Verification items for the finished model (mm, model axes). A direction names the side the tool comes from. Give positions to 0.01 mm unless a question says otherwise; leave off trailing zeros. Order: outer loops, then holes, each group sorted by start corner. A loop starts at its lowest first (then second) coordinate and runs counter-clockwise, first axis right, second up. Notation, with made-up numbers: M 7.5,-5 L 41.5,-5 A14 ccw 41.5,-1 Z; hole C -20,17.25 d5. An arc over 180 degrees is marked long. Answer as a JSON object with one key per item and string values.
```python
from build123d import *

# Parameters (mm, degrees)
F0_R     = 16
F1_DEPTH = 25
F3_R     = 7.5
F4_DEPTH = 20
F5_T     = -2
F6_R     = 3


with BuildPart() as f1:
    # F0 (on Top) → F1 (new body)
    with BuildSketch(Plane.XY):
        Circle(F0_R)
    extrude(amount=F1_DEPTH)

    # F3 (on offset) → F4 (join)
    with BuildSketch(Plane.XZ.offset(13)):
        with Locations((0, 9.9646812305)):
            Circle(F3_R)
    extrude(amount=F4_DEPTH)

    # F5
    f5_openings = [f1.faces().sort_by_distance(p)[0] for p in [
        (0, 0, 25),
        (0, -33, 9.964681),
    ]]
    offset(amount=F5_T, openings=f5_openings, kind=Kind.INTERSECTION)

    # F6
    f6_edges = [f1.edges().sort_by_distance(p)[0] for p in [
        (-16, 0, 0),
    ]]
    fillet(f6_edges, radius=F6_R)


solid = f1.part
```
Q1. Gauge pin test, flat ends, axial feed: pin 1 Ø1.5 at (x, y) = (-4.5, -0.5) entering from +Z; pin 2 Ø4 at (y, z) = (5.5, 10) entering from +X; pin 3 Ø5 at (x, z) = (-2.5, 9) entering from -Y; pin 4 Ø8 at (y, z) = (-25.5, 22) entering from -X. Record the tip position at first contact, or that the pin passes through.
Resolved:
{"pin 1": "stops at z = 2", "pin 2": "stops at x = 15.61", "pin 3": "stops at y = 13.08", "pin 4": "passes through"}
Q2. Material ranges on L1, parallel to Z at x = 0, y = -23.5; L2, parallel to X at y = -15, z = 9.75; L3, parallel to Y at x = 0, z = 20.25, recorded low to high.
Resolved:
{"L1": "z = 2.46 to 4.46, 15.46 to 17.46", "L2": "x = -7.5 to -5.5, 5.5 to 7.5", "L3": "y = -16 to -14, 14 to 16"}
Q3. Section check D-D on y = -27.5. Record the cut outline in (x, z), then the cut area to 3 significant figures.
Resolved:
{"outline": "C 0,9.96 d15; hole C 0,9.96 d11", "area": "81.7 mm²"}
Q4. Release check for a two-part mould opening along Z. For faces 1 (the face through (-7.493, -23.435, 10.294)), 2 (the face through (0, 0, 2)), 3 (the face through (5.08, -22.8, 7.86)) record: +Z half, -Z half, draft (parallel to the pull), parting line (faces both ways), or undercut.
Resolved:
{"face 1": "parting line", "face 2": "+Z half", "face 3": "undercut"}
Q5. Tool access check on faces 4 (the face through (-0.07, -14.15, 25)), 5 (the face through (7.526, 11.805, 13.339)). Record the directions out of +Z, -Z, +X, -X, +Y, -Y that give a thin tool (end or side, any length) a straight path to the whole face; none if there is none.
Resolved:
{"face 4": "+Z, +X, -X, +Y, -Y", "face 5": "+Z"}
Q6. Section check A-A on y = 0. Record the cut outline in (x, z).
Resolved:
{"outline": "M -16,3 A3 ccw -13,0 L 13,0 A3 ccw 16,3 L 16,25 L 14,25 L 14,2 L -14,2 L -14,25 L -16,25 Z"}
Q7. Section check B-B on z = 20.25. Record the cut outline in (x, y).
Resolved:
{"outline": "C 0,0 d32; hole C 0,0 d28"}
Q8. Section check C-C on z = 5.5. Record the cut outline in (x, y), then the cut area to 3 significant figures.
Resolved:
{"outline": "M -6.03,-33 L -3.21,-33 L -3.21,-13.63 A14 cw long 3.21,-13.63 L 3.21,-33 L 6.03,-33 L 6.03,-14.82 A16 ccw long -6.03,-14.82 Z", "area": "275 mm²"}
